from build123d import *

# Parameters (mm, degrees)
BOSS_EXTRUDE1_DEPTH      = 5
BOSS_EXTRUDE1_DEPTH_BACK = 8
SKETCH1_R                = 3.8
SKETCH1_R_2              = 1.6
SKETCH2_R                = 8.5
BOSS_EXTRUDE2_DEPTH      = 4
SKETCH4_R                = 1.6
CUT_EXTRUDE1_DEPTH       = 4
SKETCH5_R                = 2.5
CUT_EXTRUDE2_DEPTH       = 3


with BuildPart() as part:
    # Sketch1 → Boss-Extrude1 (new, two sides: drawn at the far end of the back side and taken through both)
    with BuildSketch(Plane.XY.offset(-BOSS_EXTRUDE1_DEPTH_BACK)):
        with Locations((-58.8, 0)):
            Circle(SKETCH1_R)
        with Locations((-58.8, 0)):
            Circle(SKETCH1_R_2, mode=Mode.SUBTRACT)
    extrude(amount=BOSS_EXTRUDE1_DEPTH + BOSS_EXTRUDE1_DEPTH_BACK)

    # Sketch2 → Boss-Extrude2 (add)
    with BuildSketch(Plane.XY.offset(5)):
        with Locations((-58.8, 0)):
            Circle(SKETCH2_R)
    extrude(amount=BOSS_EXTRUDE2_DEPTH)

    # Sketch4 → Cut-Extrude1 (cut)
    with BuildSketch(Plane(origin=(0, 0, 5), x_dir=(-1, 0, 0), z_dir=(0, 0, -1))):
        with Locations(Location((58.8, 0, 0), (0, 0, 180))):
            Circle(SKETCH4_R)
    extrude(amount=-CUT_EXTRUDE1_DEPTH, mode=Mode.SUBTRACT)

    # Sketch5 → Cut-Extrude2 (cut)
    with BuildSketch(Plane.XY.offset(9)):
        with Locations((-58.8, 0)):
            Circle(SKETCH5_R)
    extrude(amount=-CUT_EXTRUDE2_DEPTH, mode=Mode.SUBTRACT)


solid = part.part
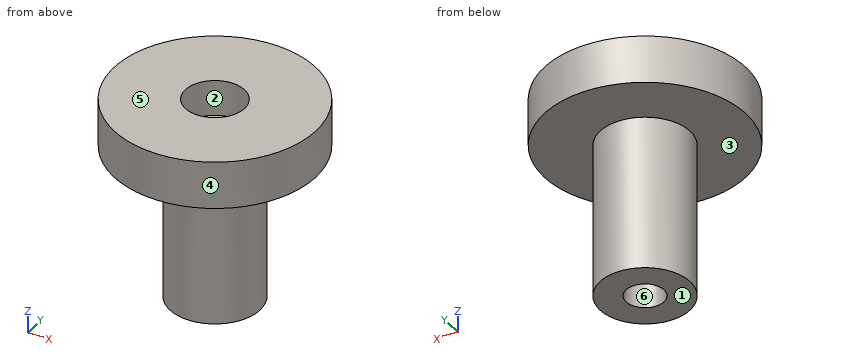
Here's how the part is built. I have some questions about the finished solid (model axes, mm). Face numbers are marked on the shaded views. A direction names the side the tool comes from. Round coordinates to 2 decimals unless told otherwise and drop trailing zeros. Write each loop counter-clockwise with the first axis right and the second up, starting at its lowest first coordinate (ties: lowest second). Pieces come first, ordered by that corner, then holes.
1. Suppose I cut it at C-C (z = 6.75). List the corners of the cut face in (x, y) for me.
2. For the marked faces 1, 2 and 3, which set-ups out of +Z, -Z, +X, -X, +Y, -Y let a thin tool reach every point of the face, with its end or its side?
3. Will these pins go through, and if not, where does the flat tip stop? pin 1 Ø3 at (x, y) = (-63, -4) entering from -Z; pin 2 Ø5 at (x, z) = (-61.5, -4) entering from +Y; pin 3 Ø1.5 at (x, y) = (-57.5, -0.5) entering from +Z; pin 4 Ø3 at (x, z) = (-53, -4) entering from +Y.
4. Suppose I cut it at D-D (x = -62.25). List the corners of the cut face in (y, z) for me.
5. I need wall thicknesses on L1, parallel to Y at x = -58.8, z = 8.1; L2, parallel to Y at x = -58.8, z = -4.25; L3, parallel to Z at x = -60.5, y = -0.5. Which ranges of each line are inside material? Lowest first, please.
6. Suppose I cut it at B-B (x = -58.8). List the corners of the cut face in (y, z) for me, and give its area (3 significant figures).
7. If we mould it in two halves opening along X, with no side actions, what happens to the marked faces 4, 5 and 6? For each: released by +X, released by -X, zero draft, split by the parting line, or undercut.
8. Suppose I cut it at A-A (y = 0). List the corners of the cut face in (x, z) for me.
Answer sheet:
1. outline: circle Ø17 at (-58.8, 0); hole circle Ø5 at (-58.8, 0)
2. face 1: -Z, +X, -X, +Y, -Y
2. face 2: +Z
2. face 3: -Z
3. pin 1: stops at z = 5
3. pin 2: stops at y = 3.79
3. pin 3: stops at z = 6
3. pin 4: passes through
4. outline: (-7.77, 5) - (-1.59, 5) - (-1.59, -8) - (1.59, -8) - (1.59, 5) - (7.77, 5) - (7.77, 9) - (-7.77, 9) - close
5. L1: y = -8.5 to -2.5, 2.5 to 8.5
5. L2: y = -3.8 to -1.6, 1.6 to 3.8
5. L3: z = -8 to 6
6. outline: (-8.5, 5) - (-3.8, 5) - (-3.8, -8) - (-1.6, -8) - (-1.6, 6) - (-2.5, 6) - (-2.5, 9) - (-8.5, 9) - close; (1.6, -8) - (3.8, -8) - (3.8, 5) - (8.5, 5) - (8.5, 9) - (2.5, 9) - (2.5, 6) - (1.6, 6) - close
6. area: 107 mm2
7. face 4: split by the parting line
7. face 5: zero draft
7. face 6: undercut
8. outline: (-67.3, 5) - (-62.6, 5) - (-62.6, -8) - (-60.4, -8) - (-60.4, 6) - (-61.3, 6) - (-61.3, 9) - (-67.3, 9) - close; (-57.2, -8) - (-55, -8) - (-55, 5) - (-50.3, 5) - (-50.3, 9) - (-56.3, 9) - (-56.3, 6) - (-57.2, 6) - close
